from build123d import *

# Parameters (mm, degrees)
SKETCH1_R           = 2.159
BOSS_EXTRUDE1_DEPTH = 16.0782
FILLET1_R           = 2.54


with BuildPart() as part:
    # Sketch1 → Boss-Extrude1 (new body)
    with BuildSketch(Plane.XY):
        with BuildLine():
            Line((0, 7.62), (76.2, 7.62))
            ThreePointArc((76.2, 7.62), (80.01, 3.81), (76.2, 0))
            Line((76.2, 0), (62.219445877, 0))
            ThreePointArc((62.219445877, 0), (53.46050014, 2.99974), (44.701554403, 0))
            Line((44.701554403, 0), (0, 0))
            ThreePointArc((0, 0), (-3.81, 3.81), (0, 7.62))
        make_face()
        with Locations((0, 3.81)):
            Circle(SKETCH1_R, mode=Mode.SUBTRACT)
        with Locations((38.1, 3.81)):
            Circle(SKETCH1_R, mode=Mode.SUBTRACT)
        with Locations((76.2, 3.81)):
            Circle(SKETCH1_R, mode=Mode.SUBTRACT)
    extrude(amount=BOSS_EXTRUDE1_DEPTH)

    # Fillet1
    fillet1_edges = [part.edges().sort_by_distance(p)[0] for p in [
        (62.219445877, 0, 8.0391),
        (44.701554403, 0, 8.0391),
    ]]
    fillet(fillet1_edges, radius=FILLET1_R)


solid = part.part
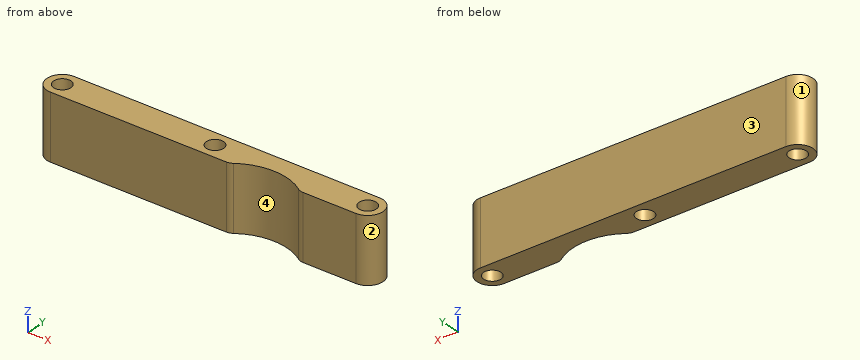
For this review, take the finished solid that the model builds, in its own axes (mm). Face numbers are marked on the shaded views. Give positions to 0.01 mm unless a question says otherwise; leave off trailing zeros. Loops run counter-clockwise (first coordinate to the right, second up) from the corner with the lowest first, then second, coordinate; pieces in that order, holes last.
Item 1: Take a section at D-D, the plane x = 75. State the section outline as (y, z) points, and give its area (3 significant figures).
Item 2: Take a section at C-C, the plane z = 1.5. State the section outline as (x, y) points (1 decimal), and give its area (3 significant figures).
Item 3: Take a section at A-A, the plane y = 3.81. State the section outline as (x, z) points.
Item 4: Draft analysis for pull direction X (two halves, no side actions). For the marked faces 1, 2, 3 and 4, state which applies: +X half, -X half, draft (parallel to the pull), parting line (faces both ways), or undercut.
Item 5: For line 1 along Y through (x, z) = (38.1, 9); line 2 along X through (y, z) = (5.75, 4); line 3 along X through (y, z) = (2, 3.5), list the stretches that pass through material, from the lowest coordinate up.
Item 6: Take a section at B-B, the plane x = 38.1. State the section outline as (y, z) points.
Calculated:
1. outline: (0, 0) - (2.02, 0) - (2.02, 16.08) - (0, 16.08) - close; (5.6, 0) - (7.62, 0) - (7.62, 16.08) - (5.6, 16.08) - close
1. area: 64.8 mm2
2. outline: (0, 0) - (43.9, 0) arc R2.5 ccw to (45.3, 0.5) arc R14.3 cw to (61.6, 0.5) arc R2.5 ccw to (63, 0) - (76.2, 0) arc R3.8 ccw to (76.2, 7.6) - (0, 7.6) arc R3.8 ccw to start; hole circle Ø4.3 at (0, 3.8); hole circle Ø4.3 at (38.1, 3.8); hole circle Ø4.3 at (76.2, 3.8)
2. area: 546 mm2
3. outline: (-3.81, 0) - (-2.16, 0) - (-2.16, 16.08) - (-3.81, 16.08) - close; (2.16, 0) - (35.94, 0) - (35.94, 16.08) - (2.16, 16.08) - close; (40.26, 0) - (74.04, 0) - (74.04, 16.08) - (40.26, 16.08) - close; (78.36, 0) - (80.01, 0) - (80.01, 16.08) - (78.36, 16.08) - close
4. face 1: -X half
4. face 2: +X half
4. face 3: draft
4. face 4: undercut
5. line 1: y = 0 to 1.65, 5.97 to 7.62
5. line 2: x = -3.28 to -0.95, 0.95 to 37.15, 39.05 to 75.25, 77.15 to 79.48
5. line 3: x = -3.35 to -1.18, 1.18 to 36.92, 39.28 to 48.21, 58.71 to 75.02, 77.38 to 79.55
6. outline: (0, 0) - (1.65, 0) - (1.65, 16.08) - (0, 16.08) - close; (5.97, 0) - (7.62, 0) - (7.62, 16.08) - (5.97, 16.08) - close
